Work out the finished part from the listing and answer in its coordinate system (mm). A direction names the side the tool comes from. Round coordinates to 2 decimals unless told otherwise and drop trailing zeros. Order: outer loops, then holes, each group sorted by start corner. A loop starts at its lowest first (then second) coordinate and runs counter-clockwise, first axis right, second up. Notation, with made-up numbers: M 3.5,-8 L 8.5,-8 A19 ccw 8.5,-2 Z; hole C -25,1 d9. An arc over 180 degrees is marked long. Return JSON: item names as keys, results as strings.
from build123d import *

# Parameters (mm, degrees)
ESQUISSE1_R                       = 5
BOSS_EXTRU_1_DEPTH                = 5
ESQUISSE2_R                       = 10
BOSS_EXTRU_2_DEPTH                = 3
ESQUISSE3_R                       = 10
BOSS_EXTRU_3_DEPTH                = 2
BOSS_EXTRU_3_DRAFT                = -50
BOSS_EXTRU_3_PROFILE_2_DEPTH      = 2
BOSS_EXTRU_3_PROFILE_2_DRAFT      = -50
BOSS_EXTRU_3_PROFILE_3_DEPTH      = 2
BOSS_EXTRU_3_PROFILE_3_DRAFT      = -50
ESQUISSE4_R                       = 12.383507185
BOSS_EXTRU_4_DEPTH                = 5
BOSS_EXTRU_4_DRAFT                = 50
BOSS_EXTRU_4_PROFILE_2_DEPTH      = 5
BOSS_EXTRU_4_PROFILE_2_DRAFT      = 50
BOSS_EXTRU_4_PROFILE_3_DEPTH      = 5
BOSS_EXTRU_4_PROFILE_3_DRAFT      = 50
ESQUISSE5_R                       = 6.424739222
BOSS_EXTRU_5_DEPTH                = 5
BOSS_EXTRU_5_DRAFT                = -50
BOSS_EXTRU_5_PROFILE_2_DEPTH      = 5
BOSS_EXTRU_5_PROFILE_2_DRAFT      = -50
BOSS_EXTRU_5_PROFILE_3_DEPTH      = 5
BOSS_EXTRU_5_PROFILE_3_DRAFT      = -50
ESQUISSE6_R                       = 9.5
ENL_V_MAT_EXTRU_1_DEPTH           = 5
ENL_V_MAT_EXTRU_1_DRAFT           = -50
ENL_V_MAT_EXTRU_1_PROFILE_2_DEPTH = 5
ENL_V_MAT_EXTRU_1_PROFILE_2_DRAFT = -50
ENL_V_MAT_EXTRU_1_PROFILE_3_DEPTH = 5
ENL_V_MAT_EXTRU_1_PROFILE_3_DRAFT = -50
ESQUISSE7_W                       = 10
ESQUISSE7_H                       = 10
ENL_V_MAT_EXTRU_2_DEPTH           = 10


with BuildPart() as part:
    # Esquisse1 → Boss.-Extru.1 (new body)
    with BuildSketch(Plane.XY):
        with BuildLine():
            Line((-98.729079498, 20), (96.270920502, 20))
            ThreePointArc((96.270920502, 20), (116.270920502, 0), (96.270920502, -20))
            Line((96.270920502, -20), (-98.729079498, -20))
            ThreePointArc((-98.729079498, -20), (-118.729079498, 0), (-98.729079498, 20))
        make_face()
        with Locations((-101.229079498, 0)):
            Circle(ESQUISSE1_R, mode=Mode.SUBTRACT)
        with Locations((-1.229079498, 0)):
            Circle(ESQUISSE1_R, mode=Mode.SUBTRACT)
        with Locations((98.770920502, 0)):
            Circle(ESQUISSE1_R, mode=Mode.SUBTRACT)
    extrude(amount=BOSS_EXTRU_1_DEPTH)

    # Esquisse2 → Boss.-Extru.2 (add)
    with BuildSketch(Plane.XY.offset(5)):
        with Locations((-101.229079498, 0)):
            Circle(ESQUISSE2_R)
        with Locations((-1.229079498, 0)):
            Circle(ESQUISSE2_R)
        with Locations((98.770920502, 0)):
            Circle(ESQUISSE2_R)
    extrude(amount=BOSS_EXTRU_2_DEPTH)


with BuildPart() as boss_extru_3_tool:
    # Esquisse3 → Boss.-Extru.3 (with draft: the straight prism first)
    with BuildSketch(Plane.XY.offset(8)):
        with Locations((-101.229079498, 0)):
            Circle(ESQUISSE3_R)
    extrude(amount=BOSS_EXTRU_3_DEPTH)
    # Boss.-Extru.3: the draft: its side faces are tilted about the plane it starts from
    boss_extru_3_sides = [boss_extru_3_tool.faces().sort_by_distance(p)[0] for p in [
        (-111.229079498, 0, 9),
    ]]
    draft(boss_extru_3_sides, Plane.XY.offset(8), BOSS_EXTRU_3_DRAFT)


with BuildPart() as part_1:
    add(part.part)

    # Boss.-Extru.3: add boss_extru_3_tool
    add(boss_extru_3_tool.part)


with BuildPart() as boss_extru_3_profile_2_tool:
    # Esquisse3 → Boss.-Extru.3 profile 2 (with draft: the straight prism first)
    with BuildSketch(Plane.XY.offset(8)):
        with Locations((-1.229079498, 0)):
            Circle(ESQUISSE3_R)
    extrude(amount=BOSS_EXTRU_3_PROFILE_2_DEPTH)
    # Boss.-Extru.3 profile 2: the draft: its side faces are tilted about the plane it starts from
    boss_extru_3_profile_2_sides = [boss_extru_3_profile_2_tool.faces().sort_by_distance(p)[0] for p in [
        (-11.229079498, 0, 9),
    ]]
    draft(boss_extru_3_profile_2_sides, Plane.XY.offset(8), BOSS_EXTRU_3_PROFILE_2_DRAFT)


with BuildPart() as part_2:
    add(part_1.part)

    # Boss.-Extru.3 profile 2: add boss_extru_3_profile_2_tool
    add(boss_extru_3_profile_2_tool.part)


with BuildPart() as boss_extru_3_profile_3_tool:
    # Esquisse3 → Boss.-Extru.3 profile 3 (with draft: the straight prism first)
    with BuildSketch(Plane.XY.offset(8)):
        with Locations((98.770920502, 0)):
            Circle(ESQUISSE3_R)
    extrude(amount=BOSS_EXTRU_3_PROFILE_3_DEPTH)
    # Boss.-Extru.3 profile 3: the draft: its side faces are tilted about the plane it starts from
    boss_extru_3_profile_3_sides = [boss_extru_3_profile_3_tool.faces().sort_by_distance(p)[0] for p in [
        (88.770920502, 0, 9),
    ]]
    draft(boss_extru_3_profile_3_sides, Plane.XY.offset(8), BOSS_EXTRU_3_PROFILE_3_DRAFT)


with BuildPart() as part_3:
    add(part_2.part)

    # Boss.-Extru.3 profile 3: add boss_extru_3_profile_3_tool
    add(boss_extru_3_profile_3_tool.part)


with BuildPart() as boss_extru_4_tool:
    # Esquisse4 → Boss.-Extru.4 (with draft: the straight prism first)
    with BuildSketch(Plane.XY.offset(10)):
        with Locations((-101.229079498, 0)):
            Circle(ESQUISSE4_R)
    extrude(amount=BOSS_EXTRU_4_DEPTH)
    # Boss.-Extru.4: the draft: its side faces are tilted about the plane it starts from
    boss_extru_4_sides = [boss_extru_4_tool.faces().sort_by_distance(p)[0] for p in [
        (-113.612586683, 0, 12.5),
    ]]
    draft(boss_extru_4_sides, Plane.XY.offset(10), BOSS_EXTRU_4_DRAFT)


with BuildPart() as part_4:
    add(part_3.part)

    # Boss.-Extru.4: add boss_extru_4_tool
    add(boss_extru_4_tool.part)


with BuildPart() as boss_extru_4_profile_2_tool:
    # Esquisse4 → Boss.-Extru.4 profile 2 (with draft: the straight prism first)
    with BuildSketch(Plane.XY.offset(10)):
        with Locations((-1.229079498, 0)):
            Circle(ESQUISSE4_R)
    extrude(amount=BOSS_EXTRU_4_PROFILE_2_DEPTH)
    # Boss.-Extru.4 profile 2: the draft: its side faces are tilted about the plane it starts from
    boss_extru_4_profile_2_sides = [boss_extru_4_profile_2_tool.faces().sort_by_distance(p)[0] for p in [
        (-13.612586683, 0, 12.5),
    ]]
    draft(boss_extru_4_profile_2_sides, Plane.XY.offset(10), BOSS_EXTRU_4_PROFILE_2_DRAFT)


with BuildPart() as part_5:
    add(part_4.part)

    # Boss.-Extru.4 profile 2: add boss_extru_4_profile_2_tool
    add(boss_extru_4_profile_2_tool.part)


with BuildPart() as boss_extru_4_profile_3_tool:
    # Esquisse4 → Boss.-Extru.4 profile 3 (with draft: the straight prism first)
    with BuildSketch(Plane.XY.offset(10)):
        with Locations((98.770920502, 0)):
            Circle(ESQUISSE4_R)
    extrude(amount=BOSS_EXTRU_4_PROFILE_3_DEPTH)
    # Boss.-Extru.4 profile 3: the draft: its side faces are tilted about the plane it starts from
    boss_extru_4_profile_3_sides = [boss_extru_4_profile_3_tool.faces().sort_by_distance(p)[0] for p in [
        (86.387413317, 0, 12.5),
    ]]
    draft(boss_extru_4_profile_3_sides, Plane.XY.offset(10), BOSS_EXTRU_4_PROFILE_3_DRAFT)


with BuildPart() as part_6:
    add(part_5.part)

    # Boss.-Extru.4 profile 3: add boss_extru_4_profile_3_tool
    add(boss_extru_4_profile_3_tool.part)


with BuildPart() as boss_extru_5_tool:
    # Esquisse5 → Boss.-Extru.5 (with draft: the straight prism first)
    with BuildSketch(Plane.XY.offset(15)):
        with Locations((-101.229079498, 0)):
            Circle(ESQUISSE5_R)
    extrude(amount=BOSS_EXTRU_5_DEPTH)
    # Boss.-Extru.5: the draft: its side faces are tilted about the plane it starts from
    boss_extru_5_sides = [boss_extru_5_tool.faces().sort_by_distance(p)[0] for p in [
        (-107.65381872, 0, 17.5),
    ]]
    draft(boss_extru_5_sides, Plane.XY.offset(15), BOSS_EXTRU_5_DRAFT)


with BuildPart() as part_7:
    add(part_6.part)

    # Boss.-Extru.5: add boss_extru_5_tool
    add(boss_extru_5_tool.part)


with BuildPart() as boss_extru_5_profile_2_tool:
    # Esquisse5 → Boss.-Extru.5 profile 2 (with draft: the straight prism first)
    with BuildSketch(Plane.XY.offset(15)):
        with Locations((-1.229079498, 0)):
            Circle(ESQUISSE5_R)
    extrude(amount=BOSS_EXTRU_5_PROFILE_2_DEPTH)
    # Boss.-Extru.5 profile 2: the draft: its side faces are tilted about the plane it starts from
    boss_extru_5_profile_2_sides = [boss_extru_5_profile_2_tool.faces().sort_by_distance(p)[0] for p in [
        (-7.65381872, 0, 17.5),
    ]]
    draft(boss_extru_5_profile_2_sides, Plane.XY.offset(15), BOSS_EXTRU_5_PROFILE_2_DRAFT)


with BuildPart() as part_8:
    add(part_7.part)

    # Boss.-Extru.5 profile 2: add boss_extru_5_profile_2_tool
    add(boss_extru_5_profile_2_tool.part)


with BuildPart() as boss_extru_5_profile_3_tool:
    # Esquisse5 → Boss.-Extru.5 profile 3 (with draft: the straight prism first)
    with BuildSketch(Plane.XY.offset(15)):
        with Locations((98.770920502, 0)):
            Circle(ESQUISSE5_R)
    extrude(amount=BOSS_EXTRU_5_PROFILE_3_DEPTH)
    # Boss.-Extru.5 profile 3: the draft: its side faces are tilted about the plane it starts from
    boss_extru_5_profile_3_sides = [boss_extru_5_profile_3_tool.faces().sort_by_distance(p)[0] for p in [
        (92.34618128, 0, 17.5),
    ]]
    draft(boss_extru_5_profile_3_sides, Plane.XY.offset(15), BOSS_EXTRU_5_PROFILE_3_DRAFT)


with BuildPart() as part_9:
    add(part_8.part)

    # Boss.-Extru.5 profile 3: add boss_extru_5_profile_3_tool
    add(boss_extru_5_profile_3_tool.part)


with BuildPart() as enl_v_mat_extru_1_tool:
    # Esquisse6 → Enlèv. mat.-Extru.1 (with draft: the straight prism first)
    with BuildSketch(Plane.XY.offset(20)):
        with Locations((-101.229079498, 0)):
            Circle(ESQUISSE6_R)
    extrude(amount=-ENL_V_MAT_EXTRU_1_DEPTH)
    # Enlèv. mat.-Extru.1: the draft: its side faces are tilted about the plane it starts from
    enl_v_mat_extru_1_sides = [enl_v_mat_extru_1_tool.faces().sort_by_distance(p)[0] for p in [
        (-110.729079498, 0, 17.5),
    ]]
    draft(enl_v_mat_extru_1_sides, Plane.XY.offset(20), ENL_V_MAT_EXTRU_1_DRAFT)


with BuildPart() as part_10:
    add(part_9.part)

    # Enlèv. mat.-Extru.1: cut by enl_v_mat_extru_1_tool
    add(enl_v_mat_extru_1_tool.part, mode=Mode.SUBTRACT)


with BuildPart() as enl_v_mat_extru_1_profile_2_tool:
    # Esquisse6 → Enlèv. mat.-Extru.1 profile 2 (with draft: the straight prism first)
    with BuildSketch(Plane.XY.offset(20)):
        with Locations((-1.229079498, 0)):
            Circle(ESQUISSE6_R)
    extrude(amount=-ENL_V_MAT_EXTRU_1_PROFILE_2_DEPTH)
    # Enlèv. mat.-Extru.1 profile 2: the draft: its side faces are tilted about the plane it starts from
    enl_v_mat_extru_1_profile_2_sides = [enl_v_mat_extru_1_profile_2_tool.faces().sort_by_distance(p)[0] for p in [
        (-10.729079498, 0, 17.5),
    ]]
    draft(enl_v_mat_extru_1_profile_2_sides, Plane.XY.offset(20), ENL_V_MAT_EXTRU_1_PROFILE_2_DRAFT)


with BuildPart() as part_11:
    add(part_10.part)

    # Enlèv. mat.-Extru.1 profile 2: cut by enl_v_mat_extru_1_profile_2_tool
    add(enl_v_mat_extru_1_profile_2_tool.part, mode=Mode.SUBTRACT)


with BuildPart() as enl_v_mat_extru_1_profile_3_tool:
    # Esquisse6 → Enlèv. mat.-Extru.1 profile 3 (with draft: the straight prism first)
    with BuildSketch(Plane.XY.offset(20)):
        with Locations((98.770920502, 0)):
            Circle(ESQUISSE6_R)
    extrude(amount=-ENL_V_MAT_EXTRU_1_PROFILE_3_DEPTH)
    # Enlèv. mat.-Extru.1 profile 3: the draft: its side faces are tilted about the plane it starts from
    enl_v_mat_extru_1_profile_3_sides = [enl_v_mat_extru_1_profile_3_tool.faces().sort_by_distance(p)[0] for p in [
        (89.270920502, 0, 17.5),
    ]]
    draft(enl_v_mat_extru_1_profile_3_sides, Plane.XY.offset(20), ENL_V_MAT_EXTRU_1_PROFILE_3_DRAFT)


with BuildPart() as part_12:
    add(part_11.part)

    # Enlèv. mat.-Extru.1 profile 3: cut by enl_v_mat_extru_1_profile_3_tool
    add(enl_v_mat_extru_1_profile_3_tool.part, mode=Mode.SUBTRACT)

    # Esquisse7 → Enlèv. mat.-Extru.2 (cut)
    with BuildSketch(Plane(origin=(0, 0, 0), x_dir=(-1, 0, 0), z_dir=(0, 0, -1))):
        with Locations((-79.770920502, -8)):
            Rectangle(ESQUISSE7_W, ESQUISSE7_H)
        Polygon((65.729079498, 20), (63.290744845, 9.096400069), (56.165717759, -0.455876038), (51.791778882, -0.455876038), (47.417840004, -0.455876038), (40.292812918, 9.096400069), (37.854478265, 20), align=None)
        with Locations((-17.770920502, -8)):
            Rectangle(ESQUISSE7_W, ESQUISSE7_H)
        with Locations((82.229079498, -8)):
            Rectangle(ESQUISSE7_W, ESQUISSE7_H)
        Polygon((-36.709255155, 9.096400069), (-43.834282241, -0.455876038), (-48.208221118, -0.455876038), (-52.582159996, -0.455876038), (-59.707187082, 9.096400069), (-62.145521735, 20), (-34.270920502, 20), align=None)
    extrude(amount=-ENL_V_MAT_EXTRU_2_DEPTH, mode=Mode.SUBTRACT)


solid = part_12.part
Item 1: Find section C-C (z = 17.75). Determine the outline of the cut face in (x, y).
Output:
{"outline": "C -101.23,0 d19.4; C -1.23,0 d19.4; C 98.77,0 d19.4; hole C -101.23,0 d13.64; hole C -1.23,0 d13.64; hole C 98.77,0 d13.64"}
Item 2: Each of these flat-tipped pins is pushed along its axis until it touches: pin 1 (5.5 mm diameter, centred on x = -103, y = -1, fed in from +Z); pin 2 (8 mm diameter, centred on y = 10.5, z = 7, fed in from -X); pin 3 (3 mm diameter, centred on x = 99.5, y = 1, fed in from -Z); pin 4 (4 mm diameter, centred on y = -11, z = 14, fed in from +X). Where does it stop, or does it pass through?
Output:
{"pin 1": "stops at z = 16.04", "pin 2": "stops at x = -117.45", "pin 3": "stops at z = 5", "pin 4": "passes through"}
Item 3: Consider line 1 along X through (y, z) = (-11, 1.5); line 2 along X through (y, z) = (-2, 8); line 3 along Y through (x, z) = (83.5, 3). Determine where each line is inside the solid, lowest interval first. Write a range as [from, to].
Output:
{"line 1": "x = [-115.43, -87.23], [-77.23, 12.77], [22.77, 74.77], [84.77, 112.97]", "line 2": "x = [-111.03, -91.43], [-11.03, 8.57], [88.97, 108.57]", "line 3": "y = [-20, -13], [-3, 20]"}
Item 4: Find section B-B (y = 16). Determine the outline of the cut face in (x, z).
Output:
{"outline": "M -110.73,0 L -64.83,0 L -64.83,5 L -110.73,5 Z; M -38.75,0 L 35.17,0 L 35.17,5 L -38.75,5 Z; M 61.25,0 L 108.27,0 L 108.27,5 L 61.25,5 Z"}
Item 5: Find section D-D (x = -53.5). Determine the outline of the cut face in (y, z), plus the area to 3 significant figures.
Output:
{"outline": "M -20,0 L -0.46,0 L -0.46,5 L -20,5 Z", "area": "97.7 mm^2"}
Item 6: The mould has two halves that part along Y. Classify faces 1 (the flat face through (-82, -13, 2)), 2 (the flat face through (-1, 0, 5)), 3 (the flat face through (0, -13, 5)), 4 (the flat face through (-43.91, 4.25, 2.46)): pulls with the +Y half, pulls with the -Y half, needs draft (parallel to the pull), parting line crosses it, or undercut.
Output:
{"face 1": "undercut", "face 2": "undercut", "face 3": "needs draft", "face 4": "pulls with the +Y half"}
Item 7: Find section A-A (z = 2.5). State how many separate pieces and enclosed holes the cut face has, plus the area to 3 significant figures.
Output:
{"separate pieces": "1", "enclosed holes": "6", "area": "7,660 mm^2"}
Item 8: Which of the six approach directions +Z, -Z, +X, -X, +Y, -Y give full straight-line access (tool end or side, diameter ignored) to faces 5 (the cylindrical face through (3.54, 1.5, 2.46)), 6 (the flat face through (35.473, 14.625, 2.465)), 7 (the flat face through (99, 0, 15)), 8 (the flat face through (12.771, -8, 2)), 9 (the cylindrical face through (-3.4, -9.76, 6.48))?
Output:
{"face 5": "-Z", "face 6": "+Z, -Z, +Y", "face 7": "+Z", "face 8": "+Z, -Z", "face 9": "none"}
